from build123d import *

# Parameters (mm, degrees)
F1_DEPTH = 100
F2_R     = 75
F3_DEPTH = 267
F4_W     = 70
F4_H     = 20
F5_DEPTH = 231


with BuildPart() as f1:
    # F0 (on Front) → F1 (new body)
    with BuildSketch(Plane.XZ):
        with BuildLine():
            Line((120, 175), (-120, 175))
            ThreePointArc((-120, 175), (-123.535534, 173.535534), (-125, 170))
            Line((-125, 170), (-76.379128, 0))
            Line((-76.379128, 0), (-124.313403, -172.528746))
            ThreePointArc((-124.313403, -172.528746), (-122.485585, -174.338417), (-120, -175))
            Line((-120, -175), (120, -175))
            ThreePointArc((120, -175), (123.535534, -173.535534), (125, -170))
            Line((125, -170), (76.379128, 0))
            Line((76.379128, 0), (125, 170))
            ThreePointArc((125, 170), (123.535534, 173.535534), (120, 175))
        make_face()
    extrude(amount=F1_DEPTH)

    # F2 (on face) → F3 (cut)
    with BuildSketch(Plane.XZ.offset(100)):
        with Locations((0, -11.24055)):
            Circle(F2_R)
    extrude(amount=-F3_DEPTH, mode=Mode.SUBTRACT)

    # F4 (on face) → F5 (cut)
    with BuildSketch(Plane.XY.offset(175)):
        with Locations((29.123203, -60)):
            Rectangle(F4_W, F4_H)
    extrude(amount=-F5_DEPTH, mode=Mode.SUBTRACT)


solid = f1.part
Part model, mm, in its own coordinate system. A direction names the side the tool comes from. Coordinates: 2 decimals unless noted, no trailing zeros. Write each loop counter-clockwise with the first axis right and the second up, starting at its lowest first coordinate (ties: lowest second). Pieces come first, ordered by that corner, then holes. Notation, with made-up numbers: (86, -29) - (126, -29) arc R35 cw to (126, 3) - close; hole circle Ø3 at (19, 66.25). An arc over 180 degrees is marked (long way). Put each result on its own line as item: value.
1. Band-saw the part on B-B (y = -59). Write the cut outline in (x, z), then the cut area to 3 significant figures.
Final values:
outline: (-125, 170) - (-76.38, 0) - (-124.31, -172.53) arc R5 ccw to (-120, -175) - (120, -175) arc R5 ccw to (125, -170) - (76.38, 0) - (125, 170) arc R5 ccw to (120, 175) - (64.12, 175) - (64.12, 27.66) arc R75 cw to (64.12, -50.14) - (64.12, -56) - (60.18, -56) arc R75 cw (long way) to (-5.88, 63.53) - (-5.88, 175) - (-120, 175) arc R5 ccw to start
area: 44,700 mm²
2. Band-saw the part on D-D (x = -49). Write the cut outline in (y, z), then the cut area to 3 significant figures.
Final values:
outline: (-100, -175) - (0, -175) - (0, -68.02) - (-100, -68.02) - close; (-100, 45.54) - (0, 45.54) - (0, 175) - (-100, 175) - close
area: 23,600 mm²
3. Flat gauge pins, fed straight in: pin 1 Ø10 at (y, z) = (-56, 125) entering from +X; pin 2 Ø22 at (y, z) = (-63.5, 82.5) entering from -X; pin 3 Ø6 at (y, z) = (-86, 14) entering from -X; pin 4 Ø3 at (x, z) = (62.5, -52.5) entering from -Y. Where does each tip first touch, or does it go through?
Final values:
pin 1: stops at x = 113.56
pin 2: stops at x = -103.12
pin 3: stops at x = -81.24
pin 4: stops at y = -100
4. Two-plate mould, pull along X, no slides. Class faces 1 (the flat face through (-101.03, -49.3, 86.19)), 2 (the cylindrical face through (-16.259, -50.7, -84.457)), 3 (the flat face through (2, -49, 175)), 4 (the flat face through (-5.877, -60, 120)): +X half, -X half, draft (parallel to the pull), parting line (faces both ways), or undercut.
Final values:
face 1: -X half
face 2: undercut
face 3: draft
face 4: undercut
5. Band-saw the part on A-A (x = 0). Write the cut outline in (y, z).
Final values:
outline: (-100, -175) - (0, -175) - (0, -86.24) - (-100, -86.24) - close; (-100, 63.76) - (-70, 63.76) - (-70, 175) - (-100, 175) - close; (-50, 63.76) - (0, 63.76) - (0, 175) - (-50, 175) - close
6. 3-axis set-ups, long thin cutter, end or side, ignore diameter. For faces 5 (the flat face through (29, -70, 119)), 6 (the flat face through (-2, -49, -175)), 7 (the flat face through (53.8, 0, 41.3)), 8 (the flat face through (-100.01, -49.3, -85.06)), 9 (the flat face through (100.35, -49.3, 83.81)): which of +Z, -Z, +X, -X, +Y, -Y reach the whole face in a straight line?
Final values:
face 5: +Z
face 6: -Z, +X, -X, +Y, -Y
face 7: +Z, -Z, +X, -X, +Y
face 8: -X, +Y, -Y
face 9: +X, +Y, -Y
7. Probe line 1 along Y through (x, z) = (-5, 155); line 2 along Z through (x, y) = (0, -61.5); line 3 along Z through (x, y) = (0, -78). List the from-to ranges inside material, lowest first. Write a range as [from, to].
Final values:
line 1: y = [-100, -70], [-50, 0]
line 2: z = [-175, -86.24]
line 3: z = [-175, -86.24], [63.76, 175]
8. Band-saw the part on C-C (z = -76). Write the cut outline in (x, y), then the cut area to 3 significant figures.
Final values:
outline: (-97.49, -100) - (-37.83, -100) - (-37.83, 0) - (-97.49, 0) - close; (37.83, -100) - (98.12, -100) - (98.12, 0) - (37.83, 0) - close
area: 12,000 mm²
